from build123d import *

# Parameters (mm, degrees)
SKETCH1_W           = 279.4
SKETCH1_H           = 76.2
BOSS_EXTRUDE1_DEPTH = 6.35
CUT_EXTRUDE2_DEPTH  = 139.7
CUT_EXTRUDE3_DEPTH  = 38.1


with BuildPart() as part:
    # Sketch1 → Boss-Extrude1 (new, symmetric)
    with BuildSketch(Plane.XY):
        Rectangle(SKETCH1_W, SKETCH1_H)
    extrude(amount=BOSS_EXTRUDE1_DEPTH, both=True)

    # Sketch2 → Cut-Extrude2 (cut, symmetric)
    with BuildSketch(Plane(origin=(0, 0, 0), x_dir=(0, 0, -1), z_dir=(1, 0, 0))):
        Polygon((6.35, 38.1), (-6.35, 25.4), (-6.35, 38.1), align=None)
    extrude(amount=CUT_EXTRUDE2_DEPTH, both=True, mode=Mode.SUBTRACT)

    # Sketch3 → Cut-Extrude3 (cut, symmetric)
    with BuildSketch(Plane.XY):
        with BuildLine():
            Line((84.1375, -7.9375), (84.1375, 7.9375))
            ThreePointArc((84.1375, 7.9375), (88.9, 12.7), (93.6625, 7.9375))
            Line((93.6625, 7.9375), (93.6625, -7.9375))
            ThreePointArc((93.6625, -7.9375), (88.9, -12.7), (84.1375, -7.9375))
        make_face()
        with BuildLine():
            Line((-4.7625, -7.9375), (-4.7625, 7.9375))
            ThreePointArc((-4.7625, 7.9375), (0, 12.7), (4.7625, 7.9375))
            Line((4.7625, 7.9375), (4.7625, -7.9375))
            ThreePointArc((4.7625, -7.9375), (0, -12.7), (-4.7625, -7.9375))
        make_face()
        with BuildLine():
            Line((-93.6625, -7.9375), (-93.6625, 7.9375))
            ThreePointArc((-93.6625, 7.9375), (-88.9, 12.7), (-84.1375, 7.9375))
            Line((-84.1375, 7.9375), (-84.1375, -7.9375))
            ThreePointArc((-84.1375, -7.9375), (-88.9, -12.7), (-93.6625, -7.9375))
        make_face()
    extrude(amount=CUT_EXTRUDE3_DEPTH, both=True, mode=Mode.SUBTRACT)


solid = part.part
Could you check a few things on this model? Use its own coordinates, in mm. A direction names the side the tool comes from. Give positions to 0.01 mm unless a question says otherwise; leave off trailing zeros. Write each loop counter-clockwise with the first axis right and the second up, starting at its lowest first coordinate (ties: lowest second). Pieces come first, ordered by that corner, then holes. Notation, with made-up numbers: (-17, 77) -> (16, 77) arc R12 ccw to (16, 95) -> close; hole circle Ø11 at (58, 81.5). An arc over 180 degrees is marked (long way). Answer as a JSON object with one key per item and string values.
Q1. Will these pins go through, and if not, where does the flat tip stop? pin 1 Ø3 at (x, z) = (17.5, -3.5) entering from +Y; pin 2 Ø2 at (x, z) = (27, 3) entering from +Y.
Taken from the geometry:
{"pin 1": "stops at y = 36.75", "pin 2": "stops at y = 29.75"}
Q2. We'd pull the mould along X, two halves only. Please class faces 1 (the flat face through (-139.7, -1, 0)), 2 (the cylindrical face through (-89, 12.7, 0.1)), 3 (the flat face through (1.96, 31.84, -0.09)), 4 (the flat face through (-84.138, 0, 0)): released by +X, released by -X, zero draft, split by the parting line, or undercut.
Taken from the geometry:
{"face 1": "released by -X", "face 2": "undercut", "face 3": "zero draft", "face 4": "undercut"}
Q3. Which directions (+Z, -Z, +X, -X, +Y, -Y) give clear straight access to the entire face, cutting with the end or side of a thin tool? Please do faces 5 (the cylindrical face through (-88.8, -12.7, 0.1)), 6 (the flat face through (-2, 17, -6.35)).
Taken from the geometry:
{"face 5": "+Z, -Z", "face 6": "-Z, +X, -X, +Y, -Y"}
Q4. Suppose I cut it at A-A on y = 3. Write out the boundary of the cut face in (x, z), then the cut area to 3 significant figures.
Taken from the geometry:
{"outline": "(-139.7, -6.35) -> (-93.66, -6.35) -> (-93.66, 6.35) -> (-139.7, 6.35) -> close; (-84.14, -6.35) -> (-4.76, -6.35) -> (-4.76, 6.35) -> (-84.14, 6.35) -> close; (4.76, -6.35) -> (84.14, -6.35) -> (84.14, 6.35) -> (4.76, 6.35) -> close; (93.66, -6.35) -> (139.7, -6.35) -> (139.7, 6.35) -> (93.66, 6.35) -> close", "area": "3,190 mm²"}
Q5. Suppose I cut it at D-D on x = 45.5. Write out the boundary of the cut face in (y, z).
Taken from the geometry:
{"outline": "(-38.1, -6.35) -> (38.1, -6.35) -> (25.4, 6.35) -> (-38.1, 6.35) -> close"}
Q6. Please list where these lines run through material, in increasing order: L1, parallel to X at y = 4, z = 4.75; L2, parallel to X at y = 12, z = 3; L3, parallel to Z at x = -41, y = 30.
Taken from the geometry:
{"L1": "x = -139.7 to -93.66, -84.14 to -4.76, 4.76 to 84.14, 93.66 to 139.7", "L2": "x = -139.7 to -91.39, -86.41 to -2.49, 2.49 to 86.41, 91.39 to 139.7", "L3": "z = -6.35 to 1.75"}
Q7. Suppose I cut it at C-C on x = 88.9. Write out the boundary of the cut face in (y, z).
Taken from the geometry:
{"outline": "(-38.1, -6.35) -> (-12.7, -6.35) -> (-12.7, 6.35) -> (-38.1, 6.35) -> close; (12.7, -6.35) -> (38.1, -6.35) -> (25.4, 6.35) -> (12.7, 6.35) -> close"}
Q8. Suppose I cut it at B-B on z = -3.75. Write out the boundary of the cut face in (x, y) (1 decimal).
Taken from the geometry:
{"outline": "(-139.7, -38.1) -> (139.7, -38.1) -> (139.7, 35.5) -> (-139.7, 35.5) -> close; hole (-93.7, -7.9) arc R4.8 ccw to (-84.1, -7.9) -> (-84.1, 7.9) arc R4.8 ccw to (-93.7, 7.9) -> close; hole (-4.8, -7.9) arc R4.8 ccw to (4.8, -7.9) -> (4.8, 7.9) arc R4.8 ccw to (-4.8, 7.9) -> close; hole (84.1, -7.9) arc R4.8 ccw to (93.7, -7.9) -> (93.7, 7.9) arc R4.8 ccw to (84.1, 7.9) -> close"}
